Answer from the drawing. Dimensions are ordinates in mm from the lowest x, y and z of the part. A direction names the side the tool comes from. Give positions to 0.01 mm unless a question says otherwise; leave off trailing zeros. Order: outer loops, then holes, each group sorted by start corner. A loop starts at its lowest first (then second) coordinate and runs counter-clockwise, first axis right, second up. Notation, with made-up numbers: (42, 26) - (87, 26) arc R27 ccw to (87, 62) - close; hole circle Ø8 at (34.5, 89.25). An arc over 180 degrees is marked (long way). Answer in a Markdown table with one row per item. Add a question column.
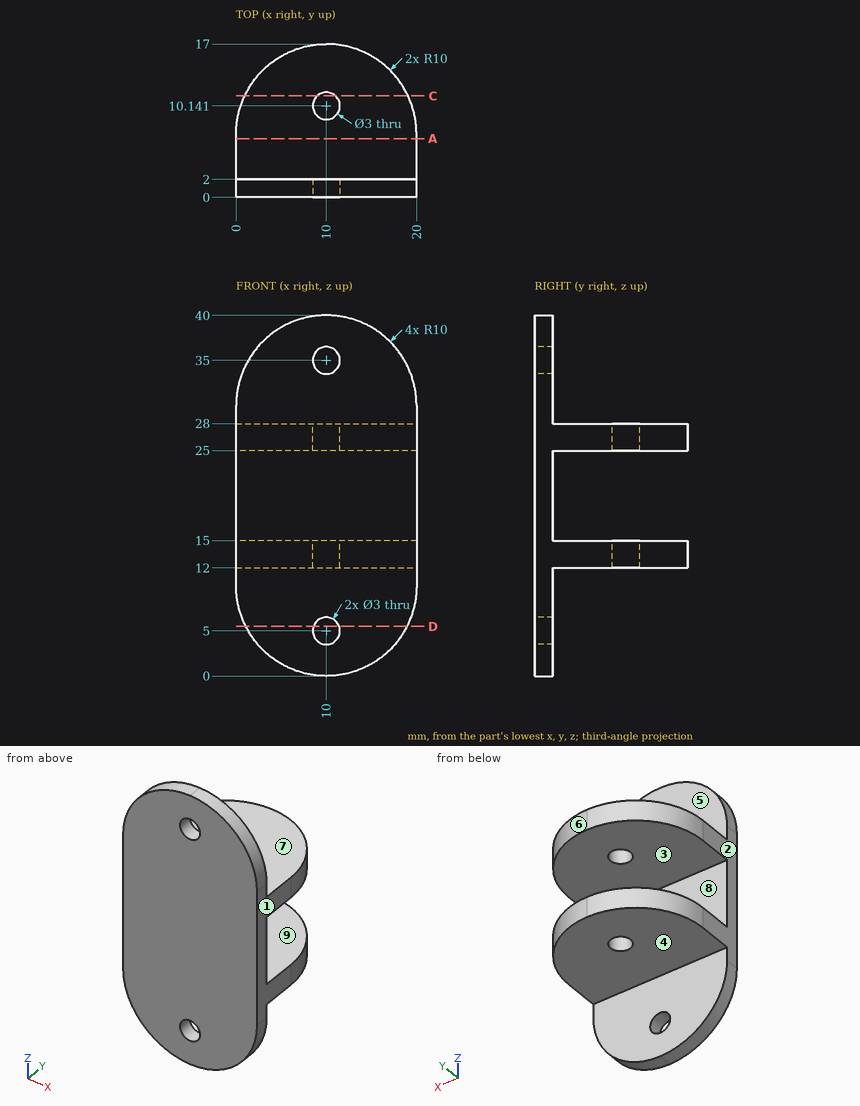
(1) Each of these flat-tipped pins is pushed along its axis until it touches: P1, Ø3.5, axis at x = 10, y = 10.14, coming from the +Z side; P2, Ø6, axis at x = 7.5, y = 12, coming from the -Z side; P3, Ø2.5, axis at x = 10, y = 10.14, coming from the +Z side; P4, Ø1, axis at x = 14.5, z = 34.5, coming from the +Y side. Where does it stop, or does it pass through?
(2) For the marked faces 1, 2, 3, 4 and 5, determine the directions among +Z, -Z, +X, -X, +Y, -Y from which every point of the face is accessible in a straight line to the end or side of a thin tool.
(3) Straight lines are drawn through the part: line 1 (Y direction, x = 10, z = 27); line 2 (Z direction, x = 10, y = 15); line 3 (Z direction, x = 10, y = 1.45). For each, find the intervals that lie inside material, in ascending order.
(4) Find section C-C, the plane y = 11.25. Write down the section's boundary in (x, z), plus the area to 3 significant figures.
(5) Find section A-A, the plane y = 6.5. Write down the section's boundary in (x, z).
(6) Find section D-D, the plane z = 5.5. Write down the section's boundary in (x, y).
(7) The mould has two halves that part along Z. Classify the marked faces 6, 7, 8 and 9: +Z half, -Z half, draft (parallel to the pull), parting line (faces both ways), or undercut.
Answer key:
| question | item | result |
|---|---|---|
| 1 | P1 | z = 28 |
| 1 | P2 | z = 12 |
| 1 | P3 | through |
| 1 | P4 | y = 2 |
| 2 | face 1 | +Z, -Z, +X, +Y, -Y |
| 2 | face 2 | +Z, -Z, -X, +Y, -Y |
| 2 | face 3 | +X, -X, +Y |
| 2 | face 4 | -Z, +X, -X, +Y |
| 2 | face 5 | +Z, +X, -X, +Y |
| 3 | line 1 | 0 to 8.64, 11.64 to 17 |
| 3 | line 2 | 12 to 15, 25 to 28 |
| 3 | line 3 | 0 to 3.5, 6.5 to 33.5, 36.5 to 40 |
| 4 | outline | (0.95, 12) - (8.99, 12) - (8.99, 15) - (0.95, 15) - close; (0.95, 25) - (8.99, 25) - (8.99, 28) - (0.95, 28) - close; (11.01, 12) - (19.05, 12) - (19.05, 15) - (11.01, 15) - close; (11.01, 25) - (19.05, 25) - (19.05, 28) - (11.01, 28) - close |
| 4 | area | 96.5 mm² |
| 5 | outline | (0, 12) - (20, 12) - (20, 15) - (0, 15) - close; (0, 25) - (20, 25) - (20, 28) - (0, 28) - close |
| 6 | outline | (1.07, 0) - (8.59, 0) - (8.59, 2) - (1.07, 2) - close; (11.41, 0) - (18.93, 0) - (18.93, 2) - (11.41, 2) - close |
| 7 | face 6 | draft |
| 7 | face 7 | +Z half |
| 7 | face 8 | undercut |
| 7 | face 9 | undercut |
